from build123d import *

# Parameters (mm, degrees)
F1_DEPTH = 450
F2_R     = 4
F3_R     = 7


with BuildPart() as f1:
    # F0 (on Front) → F1 (new body, symmetric)
    with BuildSketch(Plane.XZ):
        Polygon((-102.5, 0), (-102.5, -16), (102.5, -16), (102.5, 0), (99.5, 0), (99.5, -13), (-99.5, -13), (-99.5, 0), align=None)
    extrude(amount=F1_DEPTH, both=True)

    # F2
    f2_edges = [f1.edges().sort_by_distance(p)[0] for p in [
        (-99.5, 0, -13),
        (99.5, 0, -13),
    ]]
    fillet(f2_edges, radius=F2_R)

    # F3
    f3_edges = [f1.edges().sort_by_distance(p)[0] for p in [
        (-102.5, 0, -16),
        (102.5, 0, -16),
    ]]
    fillet(f3_edges, radius=F3_R)


solid = f1.part
Design review of the part built by this model. Coordinates are the model's own, in mm. Round coordinates to 2 decimals unless told otherwise and drop trailing zeros. Write each loop counter-clockwise with the first axis right and the second up, starting at its lowest first coordinate (ties: lowest second). Pieces come first, ordered by that corner, then holes. Notation, with made-up numbers: (84.5, -14) - (95.5, -14) arc R26 ccw to (95.5, 19) - close; hole circle Ø6 at (12.5, 57.5). An arc over 180 degrees is marked (long way). Return JSON: item names as keys, results as strings. Group by question number.
Item 1: We need section B-B on y = 324. Write out the cut boundary in (x, z).
Item 2: Insertion check: P1, Ø10, axis at x = 47.5, y = -291, coming from the +Z side. The pin has a flat end and moves straight along its axis. Give the tip position at first contact, or say it passes through.
Item 3: For probe 1 along X at (y, z) = (307.5, -9); probe 2 along Z at (x, y) = (35, -284); probe 3 along X at (y, z) = (153, -12), list the stretches that pass through material, from the lowest coordinate up. Write a range as [from, to].
Item 4: We need section C-C on x = -59.5. Write out the cut boundary in (y, z).
Item 5: We need section A-A on z = -3. Write out the cut boundary in (x, y).
Item 6: The part is to be moulded in two halves that separate along X. For faces 1 (the face through (1, -6, -13)), 2 (the face through (0, -450, -14)), say which applies: pulls with the +X half, pulls with the -X half, needs draft (parallel to the pull), parting line crosses it, or undercut.
Model answer:
{
 "1": {"outline": "(-102.5, -9) arc R7 ccw to (-95.5, -16) - (95.5, -16) arc R7 ccw to (102.5, -9) - (102.5, 0) - (99.5, 0) - (99.5, -9) arc R4 cw to (95.5, -13) - (-95.5, -13) arc R4 cw to (-99.5, -9) - (-99.5, 0) - (-102.5, 0) - close"},
 "2": {"P1": "stops at z = -13"},
 "3": {"probe 1": "x = [-102.5, -99.5], [99.5, 102.5]", "probe 2": "z = [-16, -13]", "probe 3": "x = [-101.82, -98.15], [98.15, 101.82]"},
 "4": {"outline": "(-450, -16) - (450, -16) - (450, -13) - (-450, -13) - close"},
 "5": {"outline": "(-102.5, -450) - (-99.5, -450) - (-99.5, 450) - (-102.5, 450) - close; (99.5, -450) - (102.5, -450) - (102.5, 450) - (99.5, 450) - close"},
 "6": {"face 1": "undercut", "face 2": "needs draft"}
}
